Geometry: final body of the model. Coordinates: model frame, mm. A direction names the side the tool comes from. Round coordinates to 2 decimals unless told otherwise and drop trailing zeros. Order: outer loops, then holes, each group sorted by start corner. A loop starts at its lowest first (then second) coordinate and runs counter-clockwise, first axis right, second up. Notation, with made-up numbers: (44, 80) - (103, 80) arc R22 cw to (103, 94) - close; hole circle Ø6 at (42.5, 69). An arc over 180 degrees is marked (long way). Put each result on its own line as item: value. Start each with the question number.
(1) Material intervals for L1, parallel to X at y = 82, z = 0 (3 decimals); L2, parallel to Z at x = -0.5, y = 51.5; L3, parallel to X at y = 54.5, z = 2.75, sorted ascending. Write a range as [from, to].
(2) Pin query (flat end, axial travel): P1, Ø4, axis at x = -1, y = 243.5, coming from the +Z side; P2, Ø3, axis at x = -1, y = 217.5, coming from the -Z side; P3, Ø1.5, axis at y = 79.5, z = -2.5, coming from the -X side. Return the tip coordinate at first contact, or that it passes through.
(3) Section B-B (y = 169). Output: boundary loops of the cut face in (x, z) (3 decimals), and give its area (3 significant figures).
(4) Access query for faces 1 (the face through (7, 279.4, 0)), 2 (the face through (2, 284.4, -3)). Directions: +Z, -Z, +X, -X, +Y, -Y. A direction counts if a zero-diameter tool reaches every point of the face in a straight line with its end or side. Return the directions, or none.
(5) Pull-direction query (X, two-part tool) for faces 3 (the face through (-3.86, 137.74, -5.04)), 4 (the face through (3, 0, -2)), 5 (the face through (-1.93, 140.21, -2.52)); classes: released by +X, released by -X, zero draft, split by the parting line, or undercut.
(6) Section A-A (x = 0). Output: boundary loops of the cut face in (y, z) (3 decimals), and give its area (3 significant figures).
from build123d import *

# Parameters (mm, degrees)
SKETCH1_R           = 6.35
SKETCH1_R_2         = 3.175
BOSS_EXTRUDE1_DEPTH = 279.4
SKETCH2_R           = 3.175
BOSS_EXTRUDE2_DEPTH = 5
FILLET1_R           = 0.5


with BuildPart() as part:
    # Sketch1 → Boss-Extrude1 (new body)
    with BuildSketch(Plane(origin=(0, 0, 0), x_dir=(1, 0, 0), z_dir=(0, 1, 0))):
        with Locations(Location((0, 0, 0), (0, 0, 270))):
            Circle(SKETCH1_R)
        with Locations(Location((0, 0, 0), (0, 0, 270))):
            Circle(SKETCH1_R_2, mode=Mode.SUBTRACT)
    extrude(amount=BOSS_EXTRUDE1_DEPTH)

    # Sketch2 → Boss-Extrude2 (add)
    with BuildSketch(Plane(origin=(0, 279.4, 0), x_dir=(1, 0, 0), z_dir=(0, 1, 0))):
        Polygon((-8.065583261, 0), (-4.03279163, -6.985), (4.03279163, -6.985), (8.065583261, 0), (4.03279163, 6.985), (-4.03279163, 6.985), align=None)
        with Locations(Location((0, 0, 0), (0, 0, 270))):
            Circle(SKETCH2_R, mode=Mode.SUBTRACT)
    extrude(amount=BOSS_EXTRUDE2_DEPTH)

    # Fillet1
    fillet1_edges = [part.edges().sort_by_distance(p)[0] for p in [
        (-6.049187445, 284.4, -3.4925),
        (-6.049187445, 284.4, 3.4925),
        (0, 284.4, 6.985),
        (6.049187445, 284.4, 3.4925),
        (6.049187445, 284.4, -3.4925),
        (0, 284.4, -6.985),
        (-6.049187445, 279.4, -3.4925),
        (-4.03279163, 281.9, -6.985),
        (-6.049187445, 279.4, 3.4925),
        (-8.065583261, 281.9, 0),
        (0, 279.4, 6.985),
        (-4.03279163, 281.9, 6.985),
        (6.049187445, 279.4, 3.4925),
        (4.03279163, 281.9, 6.985),
        (6.049187445, 279.4, -3.4925),
        (8.065583261, 281.9, 0),
        (0, 279.4, -6.985),
        (4.03279163, 281.9, -6.985),
    ]]
    fillet(fillet1_edges, radius=FILLET1_R)


solid = part.part
Checks:
1. L1: x = [-6.35, -3.175], [3.175, 6.35]
1. L2: z = [-6.33, -3.14], [3.14, 6.33]
1. L3: x = [-5.72, -1.59], [1.59, 5.72]
2. P1: stops at z = 6.35
2. P2: stops at z = -6.35
2. P3: stops at x = -6.1
3. outline: circle Ø12.7 at (0, 0); hole circle Ø6.35 at (0, 0)
3. area: 95.0 mm²
4. face 1: -Y
4. face 2: +Z, -Z, +X, -X, +Y
5. face 3: split by the parting line
5. face 4: zero draft
5. face 5: undercut
6. outline: (0, -6.35) - (279.4, -6.35) - (279.4, -6.485) arc R0.5 ccw to (279.9, -6.985) - (283.9, -6.985) arc R0.5 ccw to (284.4, -6.485) - (284.4, -3.175) - (0, -3.175) - close; (0, 3.175) - (284.4, 3.175) - (284.4, 6.485) arc R0.5 ccw to (283.9, 6.985) - (279.9, 6.985) arc R0.5 ccw to (279.4, 6.485) - (279.4, 6.35) - (0, 6.35) - close
6. area: 1,810 mm²
